Model file for the job. Use its own axes, mm. Round coordinates to 2 decimals unless told otherwise and drop trailing zeros. Loops run counter-clockwise (first coordinate to the right, second up) from the corner with the lowest first, then second, coordinate; pieces in that order, holes last. Notation, with made-up numbers: (-13, -1) -> (44, -1) arc R14 cw to (44, 14) -> close; hole circle Ø11 at (38.25, 59). An arc over 180 degrees is marked (long way). Use a Markdown table: item, result.
from build123d import *

# Parameters (mm, degrees)
SKETCH1_R           = 2
SKETCH1_R_2         = 1.5
BOSS_EXTRUDE1_DEPTH = 3


with BuildPart() as part:
    # Sketch1 → Boss-Extrude1 (new body)
    with BuildSketch(Plane(origin=(0, 0, 0), x_dir=(1, 0, 0), z_dir=(0, 1, 0))):
        Polygon((-44.676492644, 22.127798429), (-44.676492644, -27.087694748), (45.323507356, -27.872201571), (45.323507356, 22.127798429), align=None)
        with Locations(Location((-14.676492644, -2.872201571, 0), (0, 0, 270))):
            Circle(SKETCH1_R, mode=Mode.SUBTRACT)
        with Locations(Location((-34.676492644, -2.872201571, 0), (0, 0, 270))):
            Circle(SKETCH1_R, mode=Mode.SUBTRACT)
        with Locations(Location((15.323507356, -2.872201571, 0), (0, 0, 270))):
            Circle(SKETCH1_R, mode=Mode.SUBTRACT)
        with Locations(Location((-38.676492644, 15.884701617, 0), (0, 0, 270))):
            Circle(SKETCH1_R_2, mode=Mode.SUBTRACT)
        with Locations(Location((-38.676492644, -21.62910476, 0), (0, 0, 270))):
            Circle(SKETCH1_R_2, mode=Mode.SUBTRACT)
        with Locations(Location((39.323507356, 15.884701617, 0), (0, 0, 270))):
            Circle(SKETCH1_R_2, mode=Mode.SUBTRACT)
        with Locations(Location((39.323507356, -21.62910476, 0), (0, 0, 270))):
            Circle(SKETCH1_R_2, mode=Mode.SUBTRACT)
        with BuildLine():
            Line((-34.460456453, 15.627798429), (-18.317725118, 15.627798429))
            Line((-18.317725118, 15.627798429), (-18.317725118, 2.512167108))
            ThreePointArc((-18.317725118, 2.512167108), (-19.4329567, 1.557928187), (-20.305657768, 0.377798429))
            Line((-20.305657768, 0.377798429), (-29.047327519, 0.377798429))
            ThreePointArc((-29.047327519, 0.377798429), (-33.472098814, 3.51524201), (-38.735588684, 2.204582778))
            Line((-38.735588684, 2.204582778), (-38.735588684, 11.661258938))
            ThreePointArc((-38.735588684, 11.661258938), (-35.803620086, 12.788322495), (-34.460456453, 15.627798429))
        make_face(mode=Mode.SUBTRACT)
        with BuildLine():
            Line((-11.817725118, 15.627798429), (-11.817725118, 2.965387677))
            ThreePointArc((-11.817725118, 2.965387677), (-10.2396971, 1.878045296), (-9.047327519, 0.377798429))
            Line((-9.047327519, 0.377798429), (9.694342232, 0.377798429))
            ThreePointArc((9.694342232, 0.377798429), (10.727313279, 1.723992507), (12.073507356, 2.756963553))
            Line((12.073507356, 2.756963553), (12.073507356, 15.627798429))
            Line((12.073507356, 15.627798429), (-11.817725118, 15.627798429))
        make_face(mode=Mode.SUBTRACT)
        with BuildLine():
            Line((-8.904779675, -5.861738225), (9.550345172, -5.858938653))
            ThreePointArc((9.550345172, -5.858938653), (10.622446791, -7.361080001), (12.073507356, -8.501366696))
            Line((12.073507356, -8.501366696), (12.073507356, -21.048878052))
            Line((12.073507356, -21.048878052), (-11.817725118, -20.833017395))
            Line((-11.817725118, -20.833017395), (-11.817725118, -8.709790819))
            ThreePointArc((-11.817725118, -8.709790819), (-10.132359141, -7.519873108), (-8.904779675, -5.861738225))
        make_face(mode=Mode.SUBTRACT)
        with BuildLine():
            Line((-18.317725118, -8.25657025), (-18.317725118, -20.784452687))
            Line((-18.317725118, -20.784452687), (-32.231606076, -20.784452687))
            ThreePointArc((-32.231606076, -20.784452687), (-34.826040106, -16.392310392), (-39.79198853, -15.225537869))
            Line((-39.79198853, -15.225537869), (-39.79198853, -6.882401296))
            ThreePointArc((-39.79198853, -6.882401296), (-34.217755326, -9.355993677), (-29.047327519, -6.122201571))
            Line((-29.047327519, -6.122201571), (-20.305657768, -6.122201571))
            ThreePointArc((-20.305657768, -6.122201571), (-19.4329567, -7.30233133), (-18.317725118, -8.25657025))
        make_face(mode=Mode.SUBTRACT)
        with BuildLine():
            Line((18.573507356, 15.627798429), (18.573507356, 2.756963553))
            ThreePointArc((18.573507356, 2.756963553), (19.919701434, 1.723992507), (20.952672481, 0.377798429))
            Line((20.952672481, 0.377798429), (37.672865612, 0.377798429))
            Line((37.672865612, 0.377798429), (37.672865612, 9.597780127))
            ThreePointArc((37.672865612, 9.597780127), (34.256177793, 11.81380846), (32.828586206, 15.627798429))
            Line((32.828586206, 15.627798429), (18.573507356, 15.627798429))
        make_face(mode=Mode.SUBTRACT)
        with BuildLine():
            Line((18.573507356, -8.501366696), (18.573423049, -21.172157696))
            Line((18.573423049, -21.172157696), (32.839588836, -21.172157696))
            ThreePointArc((32.839588836, -21.172157696), (34.364481553, -17.426954943), (37.808645365, -15.308092725))
            Line((37.808645365, -15.308092725), (37.669780925, -5.854673043))
            Line((37.669780925, -5.854673043), (21.097575428, -5.857186983))
            ThreePointArc((21.097575428, -5.857186983), (20.025248813, -7.360366817), (18.573507356, -8.501366696))
        make_face(mode=Mode.SUBTRACT)
    extrude(amount=BOSS_EXTRUDE1_DEPTH)


solid = part.part
Q1. Band-saw the part on B-B, the plane z = 17. Give the cut face in (x, y).
Results list:
| item | result |
|---|---|
| outline | (-44.68, 0) -> (-34.11, 0) -> (-34.11, 3) -> (-44.68, 3) -> close; (-18.32, 0) -> (-11.82, 0) -> (-11.82, 3) -> (-18.32, 3) -> close; (12.07, 0) -> (18.57, 0) -> (18.57, 3) -> (12.07, 3) -> close; (34.76, 0) -> (45.32, 0) -> (45.32, 3) -> (34.76, 3) -> close |
Q2. Band-saw the part on D-D, the plane x = -8. Give the cut face in (y, z), plus the area to 3 significant figures.
Results list:
| item | result |
|---|---|
| outline | (0, -22.13) -> (3, -22.13) -> (3, -15.63) -> (0, -15.63) -> close; (0, -0.38) -> (3, -0.38) -> (3, 5.86) -> (0, 5.86) -> close; (0, 20.87) -> (3, 20.87) -> (3, 27.41) -> (0, 27.41) -> close |
| area | 57.8 mm² |
Q3. Band-saw the part on A-A, the plane x = -25.5. Give the cut face in (y, z).
Results list:
| item | result |
|---|---|
| outline | (0, -22.13) -> (3, -22.13) -> (3, -15.63) -> (0, -15.63) -> close; (0, -0.38) -> (3, -0.38) -> (3, 6.12) -> (0, 6.12) -> close; (0, 20.78) -> (3, 20.78) -> (3, 27.25) -> (0, 27.25) -> close |
Q4. Band-saw the part on C-C, the plane z = 10.5. Give the cut face in (x, y).
Results list:
| item | result |
|---|---|
| outline | (-44.68, 0) -> (-39.79, 0) -> (-39.79, 3) -> (-44.68, 3) -> close; (-18.32, 0) -> (-11.82, 0) -> (-11.82, 3) -> (-18.32, 3) -> close; (12.07, 0) -> (18.57, 0) -> (18.57, 3) -> (12.07, 3) -> close; (37.74, 0) -> (45.32, 0) -> (45.32, 3) -> (37.74, 3) -> close |
Q5. Flat gauge pin, fed straight in: pin 1 (1.5 mm diameter, centred on x = -3, y = 1, fed in from +Z). Where does the tip first touch, or does it go through?
Results list:
| item | result |
|---|---|
| pin 1 | stops at z = 27.46 |
Q6. Pull direction Z, two halves, no side cores. Call faces 1 (the face through (-44.676, 1, 2)), 2 (the face through (-25, 1, -0.378)), 3 (the face through (40.81, 1.48, 21.43)): released by +Z, released by -Z, zero draft, split by the parting line, or undercut.
Results list:
| item | result |
|---|---|
| face 1 | zero draft |
| face 2 | undercut |
| face 3 | undercut |
Q7. Drill centre lines: L1, parallel to X at y = 1.25, z = -6; L2, parallel to X at y = 1, z = 14; L3, parallel to Z at x = 3, y = 0.35. Where is each one in solid material? Low to high. Write a range as from..to.
Results list:
| item | result |
|---|---|
| L1 | x = -44.68..-38.74, -18.32..-11.82, 12.07..18.57, 37.67..45.32 |
| L2 | x = -44.68..-39.79, -18.32..-11.82, 12.07..18.57, 37.79..45.32 |
| L3 | z = -22.13..-15.63, -0.38..5.86, 20.97..27.5 |
